The model under review builds one solid part; all positions refer to its coordinate system, in mm. A direction names the side the tool comes from. Coordinates: 2 decimals unless noted, no trailing zeros. Loops run counter-clockwise (first coordinate to the right, second up) from the corner with the lowest first, then second, coordinate; pieces in that order, holes last. Notation, with made-up numbers: M 8.25,-22.75 L 48.25,-22.75 A22 ccw 48.25,1.25 Z; hole C -6.75,58 d11. An arc over 180 degrees is marked long. Write item = value, one per line. Start each with the question number.
Q1. Wall thickness on probe 1 along Y at (x, z) = (22.5, 0.9); probe 2 along Z at (x, y) = (4.5, 12); probe 3 along Y at (x, z) = (22, 20.5): over which ranges is each line inside the solid? List them lowest first.
Q2. Mouldability with a two-part tool opening along Z and no side actions: class faces 1 (the face through (17, 16, 0)), 2 (the face through (3.55, 7.85, 14.08)), 3 (the face through (43, 2, 2)), 4 (the face through (26, 10, 4)) as released by +Z, released by -Z, zero draft, split by the parting line, or undercut.
Q3. Clearance check with flat-ended pins moving along their axes: pin 1 Ø5.5 at (x, z) = (35, 9.5) entering from -Y; pin 2 Ø1 at (x, y) = (24.5, 6) entering from +Z; pin 3 Ø9.5 at (x, y) = (22.5, 16) entering from +Z; pin 4 Ø5.5 at (y, z) = (10, 17) entering from +X. State where each tip first meets the part, or that it passes through.
Q4. We need section D-D on x = 6. Give the boundary of the cut face in (y, z).
Q5. We need section C-C on y = 12. Give the boundary of the cut face in (x, z), and give its area (3 significant figures).
Q6. We need section B-B on x = 22.5. Give the boundary of the cut face in (y, z).
Q7. For faces 5 (the face through (26, 32, 11)), 6 (the face through (10, 23, 13)), list the 3-axis set-ups (+Z, -Z, +X, -X, +Y, -Y) from which the entire face can be reached by the end or side of a thin tool; tool diameter is ignored.
Q8. We need section A-A on z = 15. Give the boundary of the cut face in (x, y), and give its area (4 significant figures).
from build123d import *

# Parameters (mm, degrees)
ESQUISSE1_W                  = 45
ESQUISSE1_H                  = 32
BOSS_EXTRU_1_DEPTH           = 22
ESQUISSE2_R                  = 5.25
ENL_V_MAT_EXTRU_1_DEPTH      = 60.439044407
ENL_V_MAT_EXTRU_2_DEPTH      = 60.439044407
ENL_V_MAT_EXTRU_2_DEPTH_BACK = 60.439044407
ESQUISSE3_R                  = 4.25
ESQUISSE4_W                  = 18
ESQUISSE4_H                  = 26
ENL_V_MAT_EXTRU_3_DEPTH      = 38
CHANFREIN1_SIZE              = 8
BOSS_EXTRU_2_DEPTH           = 18
CHANFREIN2_SIZE              = 4


with BuildPart() as part:
    # Esquisse1 → Boss.-Extru.1 (new body)
    with BuildSketch(Plane.XY):
        with Locations((22.5, 16)):
            Rectangle(ESQUISSE1_W, ESQUISSE1_H)
    extrude(amount=BOSS_EXTRU_1_DEPTH)

    # Esquisse2 → Enlèv. mat.-Extru.1 (cut, through all)
    with BuildSketch(Plane.XY.offset(22)):
        with Locations((22.5, 16)):
            Circle(ESQUISSE2_R)
    extrude(amount=-ENL_V_MAT_EXTRU_1_DEPTH, mode=Mode.SUBTRACT)

    # Esquisse3 → Enlèv. mat.-Extru.2 (cut, two sides: drawn at the far end of the back side and taken through both)
    with BuildSketch(Plane.ZY.offset(-ENL_V_MAT_EXTRU_2_DEPTH_BACK)):
        with Locations((15, 12)):
            Circle(ESQUISSE3_R)
    extrude(amount=ENL_V_MAT_EXTRU_2_DEPTH + ENL_V_MAT_EXTRU_2_DEPTH_BACK, mode=Mode.SUBTRACT)

    # Esquisse4 → Enlèv. mat.-Extru.3 (cut)
    with BuildSketch(Plane(origin=(45, 0, 0), x_dir=(0, 0, -1), z_dir=(1, 0, 0))):
        with Locations((-13, 13)):
            Rectangle(ESQUISSE4_W, ESQUISSE4_H)
    extrude(amount=-ENL_V_MAT_EXTRU_3_DEPTH, mode=Mode.SUBTRACT)

    # Chanfrein1
    chanfrein1_edges = [part.edges().sort_by_distance(p)[0] for p in [
        (45, 29, 22),
        (3.5, 0, 22),
        (0, 32, 11),
    ]]
    chamfer(chanfrein1_edges, length=CHANFREIN1_SIZE)

    # Esquisse7 → Boss.-Extru.2 (add)
    with BuildSketch(Plane.XY.offset(22)):
        Polygon((7, 26), (13, 26), (7, 20), align=None)
    extrude(amount=-BOSS_EXTRU_2_DEPTH)

    # Chanfrein2
    chanfrein2_edges = [part.edges().sort_by_distance(p)[0] for p in [
        (45, 0, 2),
    ]]
    chamfer(chanfrein2_edges, length=CHANFREIN2_SIZE)


solid = part.part
Returned:
q1.probe_1 = 0 to 10.75, 21.25 to 32
q1.probe_2 = 0 to 10.75, 19.25 to 22
q1.probe_3 = 26 to 32
q2.face_1 = released by -Z
q2.face_2 = undercut
q2.face_3 = zero draft
q2.face_4 = released by +Z
q3.pin_1 = 26
q3.pin_2 = 4
q3.pin_3 = through
q3.pin_4 = 7
q4.outline = M 0,0 L 30,0 L 30,22 L 8,22 L 0,14 Z; hole C 12,15 d8.5
q5.outline = M 0,0 L 19.1,0 L 19.1,4 L 7,4 L 7,10.75 L 0,10.75 Z; M 0,19.25 L 7,19.25 L 7,22 L 0,22 Z; M 25.9,0 L 45,0 L 45,4 L 25.9,4 Z
q5.area = 219 mm^2
q6.outline = M 0,0 L 10.75,0 L 10.75,4 L 0,4 Z; M 21.25,0 L 32,0 L 32,22 L 26,22 L 26,4 L 21.25,4 Z
q7.face_5 = +Z, -Z, +X, -X, +Y
q7.face_6 = +Z, +X, -Y
q8.outline = M 0,1 L 7,1 L 7,7.75 L 0,7.75 Z; M 0,16.25 L 7,16.25 L 7,20 L 13,26 L 44,26 L 44,32 L 8,32 L 0,24 Z
q8.area = 365.5 mm^2
